CAD build for the part. Positions are in the model's coordinates, mm. Face numbers are marked on the shaded views. A direction names the side the tool comes from. Coordinates: 2 decimals unless noted, no trailing zeros. Order: outer loops, then holes, each group sorted by start corner. A loop starts at its lowest first (then second) coordinate and runs counter-clockwise, first axis right, second up. Notation, with made-up numbers: (7, 85) -> (40, 85) arc R29 ccw to (40, 114) -> close; hole circle Ø2 at (81, 76). An arc over 180 degrees is marked (long way). Use one line per item in the form item = value. Start each with the question number.
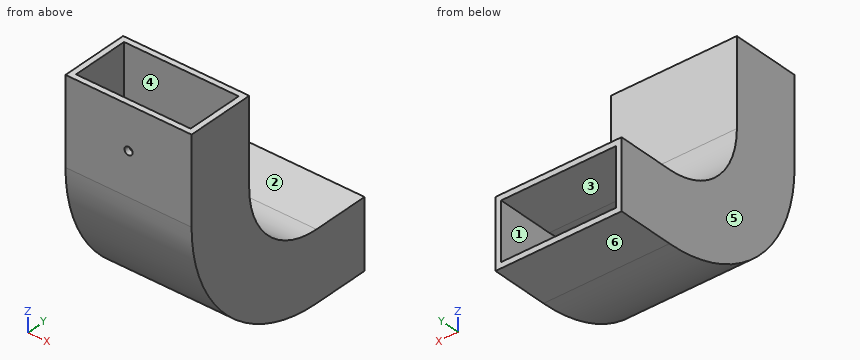
Autodesk Inventor part; units mm, degrees
ref_plane "YZ Plane" through (0, 0, 0) normal (1, 0, 0) x (0, 1, 0)
ref_plane "XZ Plane" through (0, 0, 0) normal (0, 1, 0) x (-1, 0, 0)
ref_plane "XY Plane" through (0, 0, 0) normal (0, 0, 1) x (1, 0, 0)
sketch "Sketch2" plane through (0, 0, 0) normal (0, 0, 1) x (1, 0, 0)
  line L0 (-50, -25) -> (50, -25)
  line L1 (50, -25) -> (50, 25)
  line L2 (50, 25) -> (-50, 25)
  line L3 (-50, 25) -> (-50, -25)
  line L4 (-50, -25) -> (50, 25) construction
  line L5 (50, -25) -> (-50, 25) construction
  line L6 (-55, -30) -> (55, -30)
  line L7 (55, -30) -> (55, 30)
  line L8 (55, 30) -> (-55, 30)
  line L9 (-55, 30) -> (-55, -30)
  line L10 (-55, -30) -> (55, 30) construction
  line L11 (55, -30) -> (-55, 30) construction
  point P0 (0, 0)
  dimension "d0" = 100
  dimension "d1" = 50
  dimension "d2" = 110
  dimension "d3" = 60
sketch "Sketch3" plane through (0, 0, 0) normal (1, 0, 0) x (0, 1, 0)
  line L0 (0, 0) -> (0, -75)
  arc A0 (0, -75) -> (100, -175) centre (100, -75) ccw
  line L1 (100, -75) -> (100, -175) construction
  line L2 (100, -75) -> (0, -75) construction
  line L3 (100, -175) -> (150, -175)
sweep "Sweep1" add profiles "Sketch2" path "Sketch3"
sketch "Sketch4" plane through (-55, -30, 0) normal (0, -1, 0) x (1, 0, 0)
  circle A0 centre (55, -37.5) radius 3.5
  point P0 (55, 0)
  dimension "d9" = 7
extrude "Extrusion1" cut sketch "Sketch4" against normal blind 10
properties part number "RecTubeNewTapping"
1) Cut at B-B on y = 132.5. Give the cut face in (x, z), then the cut area to 3 significant figures.
2) Drop flat-ended pins along their axis: P1, Ø10, axis at x = 25.5, y = 36, coming from the -Z side; P2, Ø6, axis at x = 21.5, y = -1, coming from the +Z side; P3, Ø10, axis at x = 39.5, y = 49.5, coming from the +Z side. Give the stop position or say it passes through.
3) Cut at C-C on z = -138.5. Give the cut face in (x, y), then the cut area to 3 significant figures.
4) Two-plate mould, pull along X, no slides. Class the marked faces 4, 5 and 6: released by +X, released by -X, zero draft, split by the parting line, or undercut.
5) Cut at A-A on x = -10.5. Give the cut face in (y, z).
6) Cut at D-D on z = -37.5. Give the cut face in (x, y).
7) 3-axis set-ups, long thin cutter, end or side, ignore diameter. For the marked faces 1, 2 and 3: which of +Z, -Z, +X, -X, +Y, -Y reach the whole face in a straight line?
8) Probe L1, parallel to Y at x = -48, z = -60; L2, parallel to X at y = 85, z = -195.5; L3, parallel to Z at x = -23.5, y = 110.5. List the from-to ranges inside material, lowest first.
Values follow:
q1.outline = (-55, -205) -> (55, -205) -> (55, -145) -> (-55, -145) -> close; hole (-50, -200) -> (50, -200) -> (50, -150) -> (-50, -150) -> close
q1.area = 1,600 mm^2
q2.P1 = -190.84
q2.P2 = -144.35
q2.P3 = -117.66
q3.outline = (-55, -13.44) -> (55, -13.44) -> (55, 70.54) -> (-55, 70.54) -> close; hole (-50, -7.67) -> (50, -7.67) -> (50, 60.09) -> (-50, 60.09) -> close
q3.area = 2,460 mm^2
q4.face_4 = undercut
q4.face_5 = released by -X
q4.face_6 = zero draft
q5.outline = (-30, -75) arc R130 ccw to (100, -205) -> (150, -205) -> (150, -200) -> (100, -200) arc R125 cw to (-25, -75) -> (-25, 0) -> (-30, 0) -> close; (25, -75) arc R75 ccw to (100, -150) -> (150, -150) -> (150, -145) -> (100, -145) arc R70 cw to (30, -75) -> (30, 0) -> (25, 0) -> close
q6.outline = (-55, -30) -> (-3.5, -30) -> (-3.5, -25) -> (-50, -25) -> (-50, 25) -> (50, 25) -> (50, -25) -> (3.5, -25) -> (3.5, -30) -> (55, -30) -> (55, 30) -> (-55, 30) -> close
q7.face_1 = none
q7.face_2 = +Z, +X, -X, +Y
q7.face_3 = +Y
q8.L1 = -30 to -25, 25 to 30
q8.L2 = -55 to -50, 50 to 55
q8.L3 = -205 to -200, -150 to -145
